Job drawing, mm, ordinate dimensions from the low corner. One solid piece. Coordinates: 2 decimals unless noted, no trailing zeros. Write each loop counter-clockwise with the first axis right and the second up, starting at its lowest first coordinate (ties: lowest second). Pieces come first, ordered by that corner, then holes. Notation, with made-up numbers: (54.5, 52) - (112.5, 52) arc R25 cw to (112.5, 73) - close; hole circle Ø4 at (-15, 35.25). An arc over 180 degrees is marked (long way). Put each result on its own line as item: value. Start each with the question number.
1. Saw through at C-C, the plane y = 6. Write the cut outline in (x, z).
2. Saw through at A-A, the plane z = 12. Write the cut outline in (x, y), plus the area to 3 significant figures.
3. Saw through at B-B, the plane x = 39. Write the cut outline in (y, z), plus the area to 3 significant figures.
4. Drill centre lines: L1, parallel to Y at x = 53.5, z = 4; L2, parallel to X at y = 8.3, z = 12; L3, parallel to Z at x = 38.5, y = 4.5. Where is each one in solid material? Low to high. Write a range as from..to.
5. Drop flat-ended pins along their axis: P1, Ø4.5, axis at x = 53.5, z = 10, coming from the +Y side; P2, Ø4.5, axis at x = 52, z = 5.5, coming from the -Y side; P3, Ø5, axis at y = 8.5, z = 6.5, coming from the +X side; P4, Ø1.8, axis at x = 52.78, z = 2, coming from the -Y side. Give the stop position or say it passes through.
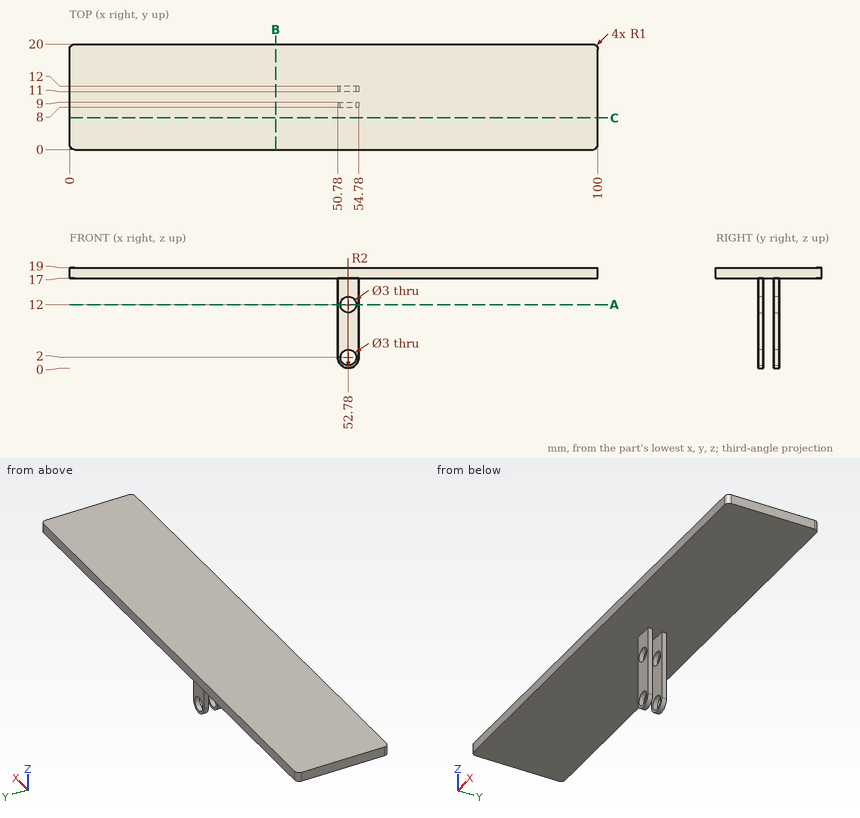
Final values:
1. outline: (0, 17) - (100, 17) - (100, 19) - (0, 19) - close
2. outline: (50.78, 8) - (51.28, 8) - (51.28, 9) - (50.78, 9) - close; (50.78, 11) - (51.28, 11) - (51.28, 12) - (50.78, 12) - close; (54.28, 8) - (54.78, 8) - (54.78, 9) - (54.28, 9) - close; (54.28, 11) - (54.78, 11) - (54.78, 12) - (54.28, 12) - close
2. area: 2.00 mm²
3. outline: (0, 17) - (20, 17) - (20, 19) - (0, 19) - close
3. area: 40.0 mm²
4. L1: y = 8..9, 11..12
4. L2: x = 50.78..51.28, 54.28..54.78
4. L3: z = 17..19
5. P1: stops at y = 12
5. P2: stops at y = 8
5. P3: stops at x = 54.78
5. P4: passes through
